The listing builds one solid part. Answer for the finished solid, in the listing's coordinates (mm). A direction names the side the tool comes from. Coordinates: 2 decimals unless noted, no trailing zeros. Order: outer loops, then holes, each group sorted by start corner. A loop starts at its lowest first (then second) coordinate and runs counter-clockwise, first axis right, second up. Notation, with made-up numbers: (47, 25) -> (85, 25) arc R18 ccw to (85, 55) -> close; hole circle Ø5 at (5.5, 38.5). An arc over 180 degrees is marked (long way). Write item = value, one per line.
from build123d import *

# Parameters (mm, degrees)
SKETCH1_W             = 45
SKETCH1_H             = 30
SKETCH1_R             = 4.32205537
BOSS_EXTRUDE1_DEPTH   = 10
M4_TAPPED_HOLE1_D     = 3.3
M4_TAPPED_HOLE1_DEPTH = 10.1
M4_TAPPED_HOLE1_TIP   = 0.991420021
CHAMFER2_SIZE         = 2


with BuildPart() as part:
    # Sketch1 → Boss-Extrude1 (new body)
    with BuildSketch(Plane.XY):
        with Locations((7.992537313, -2.5)):
            Rectangle(SKETCH1_W, SKETCH1_H)
        with Locations((22.492537313, 0.5)):
            Circle(SKETCH1_R, mode=Mode.SUBTRACT)
        with BuildLine():
            Line((-7.257462687, 5), (-7.257462687, 0))
            ThreePointArc((-7.257462687, 0), (-9.507462687, -2.25), (-11.757462687, 0))
            Line((-11.757462687, 0), (-11.757462687, 5))
            ThreePointArc((-11.757462687, 5), (-9.507462687, 7.25), (-7.257462687, 5))
        make_face(mode=Mode.SUBTRACT)
        with BuildLine():
            Line((5.742537313, 5), (5.742537313, 0))
            ThreePointArc((5.742537313, 0), (3.492537313, -2.25), (1.242537313, 0))
            Line((1.242537313, 0), (1.242537313, 5))
            ThreePointArc((1.242537313, 5), (3.492537313, 7.25), (5.742537313, 5))
        make_face(mode=Mode.SUBTRACT)
    extrude(amount=BOSS_EXTRUDE1_DEPTH)

    # M4 Tapped Hole1
    with Locations(Plane(origin=(0, 12.5, 0), x_dir=(1, 0, 0), z_dir=(0, 1, 0))):
        with Locations((22.492537313, -5)):
            Hole(M4_TAPPED_HOLE1_D / 2, depth=M4_TAPPED_HOLE1_DEPTH)
            with Locations((0, 0, -(M4_TAPPED_HOLE1_DEPTH + M4_TAPPED_HOLE1_TIP / 2))):  # 118° drill point
                Cone(0, M4_TAPPED_HOLE1_D / 2, M4_TAPPED_HOLE1_TIP, mode=Mode.SUBTRACT)

    # Chamfer2
    chamfer2_edges = [part.edges().sort_by_distance(p)[0] for p in [
        (-14.507462687, 12.5, 5),
        (30.492537313, 12.5, 5),
        (30.492537313, -17.5, 5),
        (-14.507462687, -17.5, 5),
    ]]
    chamfer(chamfer2_edges, length=CHAMFER2_SIZE)


solid = part.part
Q1. The mould has two halves that part along X. Classify faces 1 (the face through (-9.56, 7.25, 4.93)), 2 (the face through (29.507, -16.486, 4.93)), 3 (the face through (-14.507, -3, 5)): released by +X, released by -X, zero draft, split by the parting line, or undercut.
The answers:
face_1 = undercut
face_2 = released by +X
face_3 = released by -X
Q2. A tool of negligible diameter and unlimited length cuts with its end or side. For faces 4 (the face through (5.743, 3, 5)), 5 (the face through (23.802, 8.441, 6.004)), 6 (the face through (8, -2, 0)), from which of +Z, -Z, +X, -X, +Y, -Y can it reach the whole face along a straight path? Write none if from no direction.
The answers:
face_4 = +Z, -Z
face_5 = +Y
face_6 = -Z, +X, -X, +Y, -Y
Q3. Find the intervals of material crossed by line 1 along X through (y, z) = (8.5, 5); line 2 along X through (y, z) = (-0.5, 2); line 3 along X through (y, z) = (6, 8.5), in increasing order.
The answers:
line_1 = -14.51 to 20.84, 24.14 to 30.49
line_2 = -14.51 to -11.7, -7.31 to 1.3, 5.69 to 18.29, 26.7 to 30.49
line_3 = -14.51 to -11.52, -7.49 to 1.48, 5.51 to 30.49
Q4. Section D-D, the plane z = 5 is taken. Give the vertices of the cut face in (x, y).
The answers:
outline = (-14.51, -15.5) -> (-12.51, -17.5) -> (28.49, -17.5) -> (30.49, -15.5) -> (30.49, 10.5) -> (28.49, 12.5) -> (24.14, 12.5) -> (24.14, 4.49) arc R4.32 cw (long way) to (20.84, 4.49) -> (20.84, 12.5) -> (-12.51, 12.5) -> (-14.51, 10.5) -> close; hole (-11.76, 0) arc R2.25 ccw to (-7.26, 0) -> (-7.26, 5) arc R2.25 ccw to (-11.76, 5) -> close; hole (1.24, 0) arc R2.25 ccw to (5.74, 0) -> (5.74, 5) arc R2.25 ccw to (1.24, 5) -> close
Q5. Section B-B, the plane y = 3.5 is taken. Give the vertices of the cut face in (x, z).
The answers:
outline = (-14.51, 0) -> (-11.76, 0) -> (-11.76, 10) -> (-14.51, 10) -> close; (-7.26, 0) -> (1.24, 0) -> (1.24, 10) -> (-7.26, 10) -> close; (5.74, 0) -> (19.38, 0) -> (19.38, 10) -> (5.74, 10) -> close; (25.6, 0) -> (30.49, 0) -> (30.49, 10) -> (25.6, 10) -> close
Q6. This flat-tipped pin is pushed along its axis until it touches: pin 1 Ø5 at (x, y) = (22.49, 0.5) entering from +Z. Where does it stop, or does it pass through?
The answers:
pin_1 = through
Q7. Section A-A, the plane z = 2 is taken. Give the vertices of the cut face in (x, y), plus the area to 3 significant figures.
The answers:
outline = (-14.51, -15.5) -> (-12.51, -17.5) -> (28.49, -17.5) -> (30.49, -15.5) -> (30.49, 10.5) -> (28.49, 12.5) -> (-12.51, 12.5) -> (-14.51, 10.5) -> close; hole (-11.76, 0) arc R2.25 ccw to (-7.26, 0) -> (-7.26, 5) arc R2.25 ccw to (-11.76, 5) -> close; hole (1.24, 0) arc R2.25 ccw to (5.74, 0) -> (5.74, 5) arc R2.25 ccw to (1.24, 5) -> close; hole circle Ø8.64 at (22.49, 0.5)
area = 1,210 mm2
Q8. Section C-C, the plane x = -10.5 is taken. Give the vertices of the cut face in (y, z), plus the area to 3 significant figures.
The answers:
outline = (-17.5, 0) -> (-2.02, 0) -> (-2.02, 10) -> (-17.5, 10) -> close; (7.02, 0) -> (12.5, 0) -> (12.5, 10) -> (7.02, 10) -> close
area = 210 mm2
